Design review of the part shown in the three views and the two pictorial views. Dimensions are in mm from the part's minimum x, y and z. A direction names the side the tool comes from. Coordinates: 2 decimals unless noted, no trailing zeros. Order: outer loops, then holes, each group sorted by start corner. A loop starts at its lowest first (then second) coordinate and runs counter-clockwise, first axis right, second up. Notation, with made-up numbers: M 64.5,43 L 99.5,43 A19 cw 99.5,56 Z; hole C -30.5,64 d7. An arc over 180 degrees is marked long. Use CSV: the item, a comma, the result in double quotes.
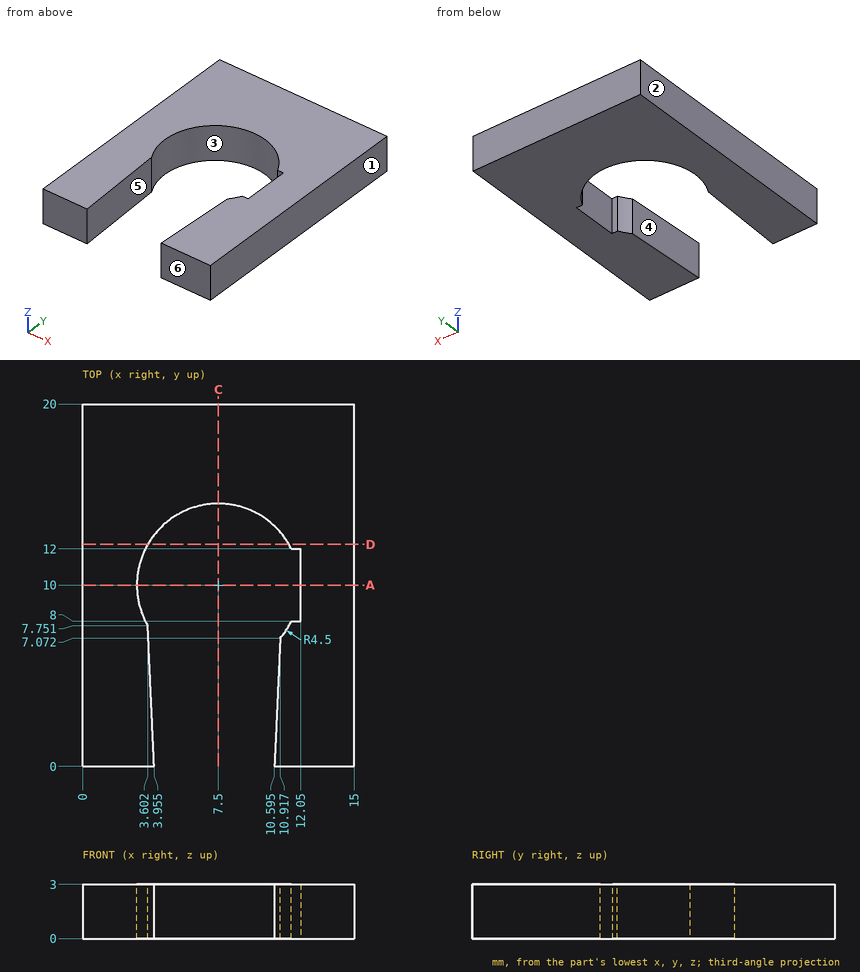
(1) Add section C-C on x = 7.5. State the section outline as (y, z) points, and give its area (3 significant figures).
The answers:
outline,"M 14.5,0 L 20,0 L 20,3 L 14.5,3 Z"
area,"16.5 mm2"
(2) Clearance check with a flat-ended pin moving along its axis: P1, Ø0.9, axis at y = 10.5, z = 1.5, coming from the -X side. State where the tip first meets the part, or that it passes through.
The answers:
P1,"stops at x = 0"
(3) Add section A-A on y = 10. State the section outline as (x, z) points.
The answers:
outline,"M 0,0 L 3,0 L 3,3 L 0,3 Z; M 12.05,0 L 15,0 L 15,3 L 12.05,3 Z"
(4) The part is to be moulded in two halves that separate along X. For the marked faces 1, 2, 3 and 4, say which applies: pulls with the +X half, pulls with the -X half, needs draft (parallel to the pull), parting line crosses it, or undercut.
The answers:
face 1,"pulls with the +X half"
face 2,"pulls with the -X half"
face 3,"undercut"
face 4,"undercut"
(5) For the marked faces 5 and 6, list the 3-axis set-ups (+Z, -Z, +X, -X, +Y, -Y) from which the entire face can be reached by the end or side of a thin tool; tool diameter is ignored.
The answers:
face 5,"+Z, -Z"
face 6,"+Z, -Z, +X, -X, -Y"
(6) Add section D-D on y = 12.25. State the section outline as (x, z) points.
The answers:
outline,"M 0,0 L 3.6,0 L 3.6,3 L 0,3 Z; M 11.4,0 L 15,0 L 15,3 L 11.4,3 Z"
(7) Wall thickness on probe 1 along X at (y, z) = (10, 1.05); probe 2 along X at (y, z) = (6.25, 2.1); probe 3 along Y at (x, z) = (9, 1.1): over which ranges is each line inside the solid? List them lowest first.
The answers:
probe 1,"x = 0 to 3, 12.05 to 15"
probe 2,"x = 0 to 3.67, 10.88 to 15"
probe 3,"y = 14.24 to 20"
